```python
from build123d import *

# Parameters (mm, degrees)
SKETCH_1_R               = 9
SKETCH_1_R_2             = 1.6
EXTRUDE_1_DEPTH          = 5
CUT_EXTRUDE_2_REACH      = 15.675
PATTERN_CIRCULAR_1_COUNT = 10
CUT_EXTRUDE_1_REACH      = 15.592
SKETCH_3_R               = 2.5
PATTERN_CIRCULAR_2_COUNT = 4


with BuildPart() as part:
    # 草图1 → 凸台-拉伸1 (new body)
    with BuildSketch(Plane(origin=(0, 0, 0), x_dir=(1, 0, 0), z_dir=(0, 1, 0))):
        with Locations(Location((0, 0, 0), (0, 0, 270))):
            Circle(SKETCH_1_R)
        with Locations(Location((0, 0, 0), (0, 0, 270))):
            Circle(SKETCH_1_R_2, mode=Mode.SUBTRACT)
    extrude(amount=EXTRUDE_1_DEPTH)

    # 草图4 → 切除-拉伸2 (cut, up to next)
    with BuildSketch(Plane(origin=(0, 5, 0), x_dir=(1, 0, 0), z_dir=(0, 1, 0)), mode=Mode.PRIVATE) as cut_extrude_2_sk1:
        with BuildLine():
            Line((-1.5, 8.874119675), (-0.599498979, 8.19962448))
            ThreePointArc((-0.599498979, 8.19962448), (0, 8), (0.599498979, 8.19962448))
            Line((0.599498979, 8.19962448), (1.5, 8.874119675))
            ThreePointArc((1.5, 8.874119675), (0, 9), (-1.5, 8.874119675))
        make_face()
    cut_extrude_2_tool1 = extrude(cut_extrude_2_sk1.sketch, amount=-CUT_EXTRUDE_2_REACH, mode=Mode.PRIVATE) & part.part
    cut_extrude_2 = cut_extrude_2_tool1.solids().sort_by_distance((0, 5, -8.590322))[0]
    add(cut_extrude_2, mode=Mode.SUBTRACT)

    # 阵列(圆周)1: 切除-拉伸2 ×10 about axis
    pattern_circular_1_axis = Axis((0, 0, 0), (0, 1, 0))
    for i in range(1, PATTERN_CIRCULAR_1_COUNT):
        add(cut_extrude_2.rotate(pattern_circular_1_axis, i * 360 / PATTERN_CIRCULAR_1_COUNT), mode=Mode.SUBTRACT)

    # 草图3 → 切除-拉伸1 (cut, up to next)
    with BuildSketch(Plane(origin=(0, 5, 0), x_dir=(1, 0, 0), z_dir=(0, 1, 0)), mode=Mode.PRIVATE) as cut_extrude_1_sk1:
        with Locations(Location((0, 5, 0), (0, 0, 270))):
            Circle(SKETCH_3_R)
    cut_extrude_1_tool1 = extrude(cut_extrude_1_sk1.sketch, amount=-CUT_EXTRUDE_1_REACH, mode=Mode.PRIVATE) & part.part
    cut_extrude_1 = cut_extrude_1_tool1.solids().sort_by_distance((0, 5, -5))[0]
    add(cut_extrude_1, mode=Mode.SUBTRACT)

    # 阵列(圆周)2: 切除-拉伸1 ×4 about axis
    pattern_circular_2_axis = Axis((0, 0, 0), (0, 1, 0))
    for i in range(1, PATTERN_CIRCULAR_2_COUNT):
        add(cut_extrude_1.rotate(pattern_circular_2_axis, i * 360 / PATTERN_CIRCULAR_2_COUNT), mode=Mode.SUBTRACT)


solid = part.part
```
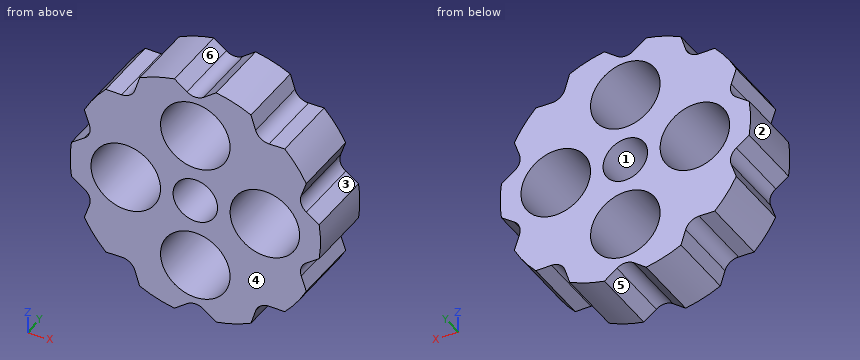
Input: part model. Units: mm. Frame: model coordinates. Face numbers are marked on the shaded views. A direction names the side the tool comes from. Round coordinates to 2 decimals unless told otherwise and drop trailing zeros. Order: outer loops, then holes, each group sorted by start corner. A loop starts at its lowest first (then second) coordinate and runs counter-clockwise, first axis right, second up. Notation, with made-up numbers: (24, -18.75) - (73, -18.75) arc R29 cw to (73, 12.25) - close; hole circle Ø9 at (-13.5, 31.25). An arc over 180 degrees is marked (long way). Answer in a Markdown table with one row per item.
Item 1: Line query: line 1 (Z direction, x = -2.25, y = 1.05); line 2 (X direction, y = 3.5, z = -1.75); line 3 (X direction, y = 3.65, z = -6.25). Output: solid intervals per line, ascending.
Model answer:
| item | result |
|---|---|
| line 1 | z = -8.71 to -6.09, -3.91 to 3.91, 6.09 to 8.71 |
| line 2 | x = -8.29 to -6.79, -3.21 to 3.21, 6.79 to 8.29 |
| line 3 | x = -6.48 to -2.17, 2.17 to 6.48 |
Item 2: Mould query, pull axis X, two halves, no side actions, for the marked faces 1, 2 and 3. Classes: released by +X, released by -X, zero draft, split by the parting line, or undercut.
Model answer:
| item | result |
|---|---|
| face 1 | undercut |
| face 2 | released by -X |
| face 3 | released by +X |
Item 3: Section query A-A (z = 0). Return the cut outline in (x, y).
Model answer:
| item | result |
|---|---|
| outline | (-9, 0) - (-7.5, 0) - (-7.5, 5) - (-9, 5) - close; (-2.5, 0) - (-1.6, 0) - (-1.6, 5) - (-2.5, 5) - close; (1.6, 0) - (2.5, 0) - (2.5, 5) - (1.6, 5) - close; (7.5, 0) - (9, 0) - (9, 5) - (7.5, 5) - close |
Item 4: Pin query (flat end, axial travel): pin 1 (3 mm diameter, centred on y = 2, z = -3.5, fed in from -X); pin 2 (2 mm diameter, centred on x = 6, y = 3.5, fed in from +Z); pin 3 (1.5 mm diameter, centred on y = 3.5, z = -5.5, fed in from +X). Return the tip coordinate at first contact, or that it passes through.
Model answer:
| item | result |
|---|---|
| pin 1 | stops at x = -7.98 |
| pin 2 | stops at z = 6.32 |
| pin 3 | stops at x = 7.64 |
Item 5: Section query B-B (x = 0). Return the cut outline in (y, z), then the cut area to 3 significant figures.
Model answer:
| item | result |
|---|---|
| outline | (0, -8) - (5, -8) - (5, -7.5) - (0, -7.5) - close; (0, -2.5) - (5, -2.5) - (5, -1.6) - (0, -1.6) - close; (0, 1.6) - (5, 1.6) - (5, 2.5) - (0, 2.5) - close; (0, 7.5) - (5, 7.5) - (5, 8) - (0, 8) - close |
| area | 14.0 mm² |
Item 6: Section query C-C (z = -2.25). Return the cut outline in (x, y), then the cut area to 3 significant figures.
Model answer:
| item | result |
|---|---|
| outline | (-7.71, 0) - (-6.09, 0) - (-6.09, 5) - (-7.71, 5) - close; (-3.91, 0) - (3.91, 0) - (3.91, 5) - (-3.91, 5) - close; (6.09, 0) - (7.71, 0) - (7.71, 5) - (6.09, 5) - close |
| area | 55.3 mm² |
Item 7: Section query D-D (x = -5). Return the cut outline in (y, z), then the cut area to 3 significant figures.
Model answer:
| item | result |
|---|---|
| outline | (0, -6.32) - (5, -6.32) - (5, -2.5) - (0, -2.5) - close; (0, 2.5) - (5, 2.5) - (5, 6.32) - (0, 6.32) - close |
| area | 38.2 mm² |
Item 8: Reachability of the marked faces 4, 5 and 6 from +Z, -Z, +X, -X, +Y, -Y: full face, straight path, thin tool, end or side. Return the list, or none.
Model answer:
| item | result |
|---|---|
| face 4 | +Z, -Z, +X, -X, -Y |
| face 5 | -Z, +Y, -Y |
| face 6 | +Z, +Y, -Y |
